Check sheet for the modelled part. Datum: model origin and axes. Units: mm. A direction names the side the tool comes from. Coordinates: 2 decimals unless noted, no trailing zeros. Loops run counter-clockwise (first coordinate to the right, second up) from the corner with the lowest first, then second, coordinate; pieces in that order, holes last. Notation, with made-up numbers: (-30, 79.25) -> (29, 79.25) arc R4 cw to (29, 84.25) -> close; hole circle Ø10 at (-26.75, 1). An arc over 180 degrees is marked (long way). Use one line per item in the form item = value.
Autodesk Inventor part; units mm, degrees
ref_plane "YZ Plane" through (0, 0, 0) normal (1, 0, 0) x (0, 1, 0)
ref_plane "XZ Plane" through (0, 0, 0) normal (0, 1, 0) x (-1, 0, 0)
ref_plane "XY Plane" through (0, 0, 0) normal (0, 0, 1) x (1, 0, 0)
sketch "Esboço1" plane through (0, 0, 0) normal (0, 0, 1) x (1, 0, 0)
  line L0 (0, 0) -> (107, 0)
  line L1 (0, 0) -> (0, 5)
  line L2 (0, 5) -> (73, 5)
  line L3 (73, 5) -> (73, 8)
  line L4 (73, 8) -> (78, 8)
  line L5 (78, 8) -> (78, 6.5)
  line L6 (78, 6.5) -> (90, 6.5)
  line L7 (90, 6.5) -> (90, 8)
  line L8 (90, 8) -> (105, 8)
  arc A0 (107, 0) -> (105, 8) centre (90, 0) ccw
  dimension "d0" = 107
  dimension "d2" = 73
  dimension "d4" = 5
  dimension "d6" = 12
  dimension "d8" = 15
  dimension "d9" = 10
  dimension "d10" = 16
  dimension "d11" = 13
  dimension "d12" = 16
revolve "Revolução1" add sketch "Esboço1" angle 360 about axis through (0, 0, 0) along (1, 0, 0)
thread "Rosca1"
sketch "Esboço2" plane through (0, 0, 0) normal (0, 0, 1) x (1, 0, 0)
  circle A0 centre (98, 0) radius 3.25
  line L0 (0, -5) -> (0, 5)
  line L1 (0, 5) -> (73, 5)
  line L2 (73, 5) -> (73, 8)
  line L3 (73, 8) -> (78, 8)
  line L4 (78, 8) -> (78, 6.5)
  line L5 (78, 6.5) -> (90, 6.5)
  line L6 (90, 6.5) -> (90, 8)
  line L7 (90, 8) -> (105, 8)
  arc A1 (105, -8) -> (105, 8) centre (90, 0) ccw
  line L8 (105, -8) -> (90, -8)
  line L9 (90, -8) -> (90, -6.5)
  line L10 (90, -6.5) -> (78, -6.5)
  line L11 (78, -6.5) -> (78, -8)
  line L12 (78, -8) -> (73, -8)
  line L13 (73, -8) -> (73, -5)
  line L14 (73, -5) -> (0, -5)
  point P0 (0, 0)
  dimension "d16" = 6.5
  dimension "d17" = 7
extrude "Extrusão1" cut sketch "Esboço2" along normal through all both and the other way through all contours A0
properties part number "Parafuso1"
(1) Mould release check, pull along Y, two halves, no side actions. Record for faces 4 (the cylindrical face through (97.6, 7.39, -3.06)), 5 (the flat face through (73, -0.1, -5.2)), 6 (the cylindrical face through (94.753, -0.143, -0.112)): +Y half, -Y half, draft (parallel to the pull), parting line (faces both ways), or undercut.
Established:
face_4 = parting line
face_5 = draft
face_6 = undercut
(2) Section check D-D, the plane x = 98. Record the boundary of the cut face in (y, z), plus the area to 4 significant figures.
Established:
outline = (-3.25, -7.31) -> (-3.25, 7.31) arc R8 ccw to start; (3.25, -7.31) arc R8 ccw to (3.25, 7.31) -> close
area = 100.0 mm²
(3) Section check A-A, the plane y = 0. Record the boundary of the cut face in (x, z), plus the area to 3 significant figures.
Established:
outline = (0, -5) -> (73, -5) -> (73, -8) -> (78, -8) -> (78, -6.5) -> (90, -6.5) -> (90, -8) -> (94.75, -8) -> (94.75, 8) -> (90, 8) -> (90, 6.5) -> (78, 6.5) -> (78, 8) -> (73, 8) -> (73, 5) -> (0, 5) -> close; (101.25, -8) -> (105, -8) arc R17 ccw to (105, 8) -> (101.25, 8) -> close
area = 1,120 mm²
(4) Section check C-C, the plane x = 80. Record the boundary of the cut face in (y, z), plus the area to 3 significant figures.
Established:
outline = circle Ø13 at (0, 0)
area = 133 mm²
(5) Section check B-B, the plane z = 0. Record the boundary of the cut face in (x, y).
Established:
outline = (0, -5) -> (73, -5) -> (73, -8) -> (78, -8) -> (78, -6.5) -> (90, -6.5) -> (90, -8) -> (105, -8) arc R17 ccw to (105, 8) -> (90, 8) -> (90, 6.5) -> (78, 6.5) -> (78, 8) -> (73, 8) -> (73, 5) -> (0, 5) -> close; hole circle Ø6.5 at (98, 0)
(6) Scan lines: line 1 along X through (y, z) = (0, -0.75); line 2 along Y through (x, z) = (98, -0.25); line 3 along X through (y, z) = (0, 4.75). Record each from-to range of solid material in increasing order.
Established:
line_1 = 0 to 94.75, 101.25 to 106.98
line_2 = -8 to -3.25, 3.25 to 8
line_3 = 0 to 94.75, 101.25 to 106.32
(7) Go/stop test with flat-tipped pins: P1, Ø3, axis at x = 64.5, z = 5.5, coming from the +Y side; P2, Ø3, axis at x = 11.5, z = 4, coming from the +Y side; P3, Ø6, axis at x = 65.5, y = 0.5, coming from the +Z side. Record where each tip stops, or that it passes through.
Established:
P1 = 3
P2 = 4.33
P3 = 5
(8) Tool access check on faces 1 (the cylindrical face through (37.01, -1.08, -4.88)), 2 (the flat face through (78, 0, 7)), 3 (the flat face through (0, 0, 0)). Record the directions out of +Z, -Z, +X, -X, +Y, -Y that give a thin tool (end or side, any length) a straight path to the whole face; none if there is none.
Established:
face_1 = -X
face_2 = none
face_3 = +Z, -Z, -X, +Y, -Y
